Check sheet for the modelled part. Datum: model origin and axes. Units: mm. Face numbers are marked on the shaded views. A direction names the side the tool comes from. Round coordinates to 2 decimals unless told otherwise and drop trailing zeros. Order: outer loops, then holes, each group sorted by start corner. A loop starts at its lowest first (then second) coordinate and runs counter-clockwise, first axis right, second up.
(1) Sectioned sample at B-B, the plane y = 12.5. Enter the section's corners in (x, z), and give its area (3 significant figures).
(2) Sectioned sample at A-A, the plane z = 4.8. Enter the section's corners in (x, y).
(3) Depth check by flat-ended pin: pin 1 (3 mm diameter, centred on x = 5, z = 4.8, fed in from +Y); pin 2 (2 mm diameter, centred on x = 10.5, y = 13.5, fed in from +Z); pin 3 (2 mm diameter, centred on x = 14.5, y = 15, fed in from -Z). Enter the tip coordinate at first touch or a pass-through.
(4) Thickness scan on probe 1 along Y at (x, z) = (12.5, 1.65); probe 2 along Z at (x, y) = (15, 1.05); probe 3 along Y at (x, z) = (3, 5.75). Record the ranges inside material, lowest first.
(5) Tool access check on the marked faces 1, 2 and 3. Record the directions out of +Z, -Z, +X, -X, +Y, -Y that give a thin tool (end or side, any length) a straight path to the whole face; none if there is none.
(6) Sectioned sample at C-C, the plane x = 5. Enter the section's corners in (y, z).
(7) Mould release check, pull along Y, two halves, no side actions. Record for the marked faces 4, 5, 6 and 7: released by +Y, released by -Y, zero draft, split by the parting line, or undercut.
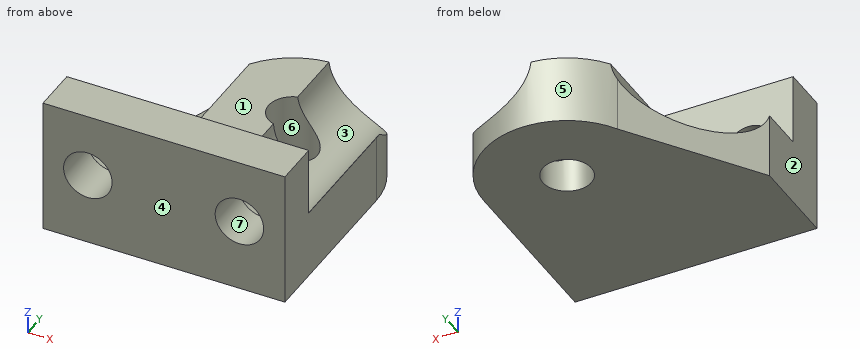
Autodesk Inventor part; units mm, degrees
ref_plane "YZ Plane" through (0, 0, 0) normal (1, 0, 0) x (0, 1, 0)
ref_plane "XZ Plane" through (0, 0, 0) normal (0, 1, 0) x (-1, 0, 0)
ref_plane "XY Plane" through (0, 0, 0) normal (0, 0, 1) x (1, 0, 0)
sketch "Sketch1" plane through (0, 0, 0) normal (0, 0, 1) x (1, 0, 0)
  circle A0 centre (12.5, 11.5) radius 1.6
  line L0 (0, 0) -> (18, 0)
  line L1 (0, 0) -> (0, 3)
  arc A1 (18, 11.5) -> (7.7369, 14.25) centre (12.5, 11.5) ccw
  line L2 (12.5, 11.5) -> (7.7369, 14.25) construction
  line L3 (12.5, 11.5) -> (18, 11.5) construction
  line L4 (7.7369, 14.25) -> (0, 3)
  line L5 (18, 11.5) -> (18, 0)
  dimension "d17" = 3
  dimension "d19" = 11.5
  dimension "d23" = 90
  dimension "d25" = 12.5
  dimension "d31" = 5.5
  dimension "d32" = 150
  dimension "d49" = 3.2
extrude "Extrusion1" add sketch "Sketch1" along normal blind 4.5
sketch "Sketch4" plane through (0, 0, 4.5) normal (0, 0, 1) x (1, 0, 0)
  line L0 (0, 3) -> (0, 0)
  line L1 (18, 0) -> (18, 3)
  line L2 (0, 0) -> (18, 0)
  line L3 (18, 0) -> (18, 3)
  line L4 (18, 3) -> (0, 3)
  line L5 (0, 3) -> (0, 0)
  line L6 (18, 0) -> (18, 11.5)
extrude "Extrusion2" add sketch "Sketch4" along normal blind 4.5
sketch "Sketch5" plane through (0, 0, 0) normal (0, -1, 0) x (1, 0, 0)
  circle A0 centre (5, 4.8) radius 1.6
  circle A1 centre (15, 4.8) radius 1.6
  line L0 (0, 0) -> (18, 0)
  point P0 (20.0001, 0)
  dimension "d13" = 3.2
  dimension "d14" = 3.2
  dimension "d38" = 4.8
  dimension "d39" = 4.8
extrude "Extrusion3" cut sketch "Sketch5" against normal through all
sketch "Sketch6" plane through (0, 3, 9) normal (0, 1, 0) x (1, 0, 0)
  circle A0 centre (5, 4.2) radius 1.6
  circle A1 centre (5, 4.2) radius 3
  circle A2 centre (15, 4.2) radius 1.6
  circle A3 centre (15, 4.2) radius 3
  line L0 (0, 9) -> (18, 9)
  point P0 (20.0001, 9)
  dimension "d34" = 6
  dimension "d35" = 6
  dimension "d40" = 4.8
  dimension "d41" = 4.8
extrude "Extrusion4" cut sketch "Sketch6" along normal up to next
sketch "Sketch7" plane through (0, 0, 0) normal (0, -1, 0) x (1, 0, 0)
  line L0 (0, 0) -> (0, 9)
  line L1 (2.042, 0) -> (0, 0)
  line L2 (0, 0) -> (0, 9)
  line L3 (0, 9) -> (2.042, 9)
  line L4 (2.042, 9) -> (2.042, 0)
extrude "Extrusion5" cut sketch "Sketch7" against normal up to next
properties part number "lower_deck_shaft_mount_v3_printing_inna_plaszczyzna_jako_baza"
Derived:
1. outline: (6.53, 0) - (11.25, 0) - (11.25, 4.5) - (7.98, 4.5) arc R3 cw to (6.53, 2.22) - close; (13.75, 0) - (17.91, 0) - (17.91, 4.06) arc R3 cw to (13.75, 2.07) - close
1. area: 28.3 mm2
2. outline: (2.04, 0) - (3.4, 0) - (3.4, 3) - (2.04, 3) - close; (6.6, 0) - (13.4, 0) - (13.4, 3) - (6.6, 3) - close; (16.6, 0) - (18, 0) - (18, 3) - (16.6, 3) - close
3. pin 1: passes through
3. pin 2: stops at z = 4.5
3. pin 3: stops at z = 0
4. probe 1: y = 0 to 9.9, 13.1 to 17
4. probe 2: z = 0 to 3.2, 6.4 to 9
4. probe 3: y = 0 to 3
5. face 1: +Z, +X, -X, +Y
5. face 2: +Z, -Z, -X, +Y, -Y
5. face 3: +Z, +Y
6. outline: (0, 0) - (10.27, 0) - (10.27, 1.8) - (3, 1.8) - (3, 3.2) - (0, 3.2) - close; (0, 6.4) - (3, 6.4) - (3, 9) - (0, 9) - close
7. face 4: released by -Y
7. face 5: released by +Y
7. face 6: undercut
7. face 7: zero draft
